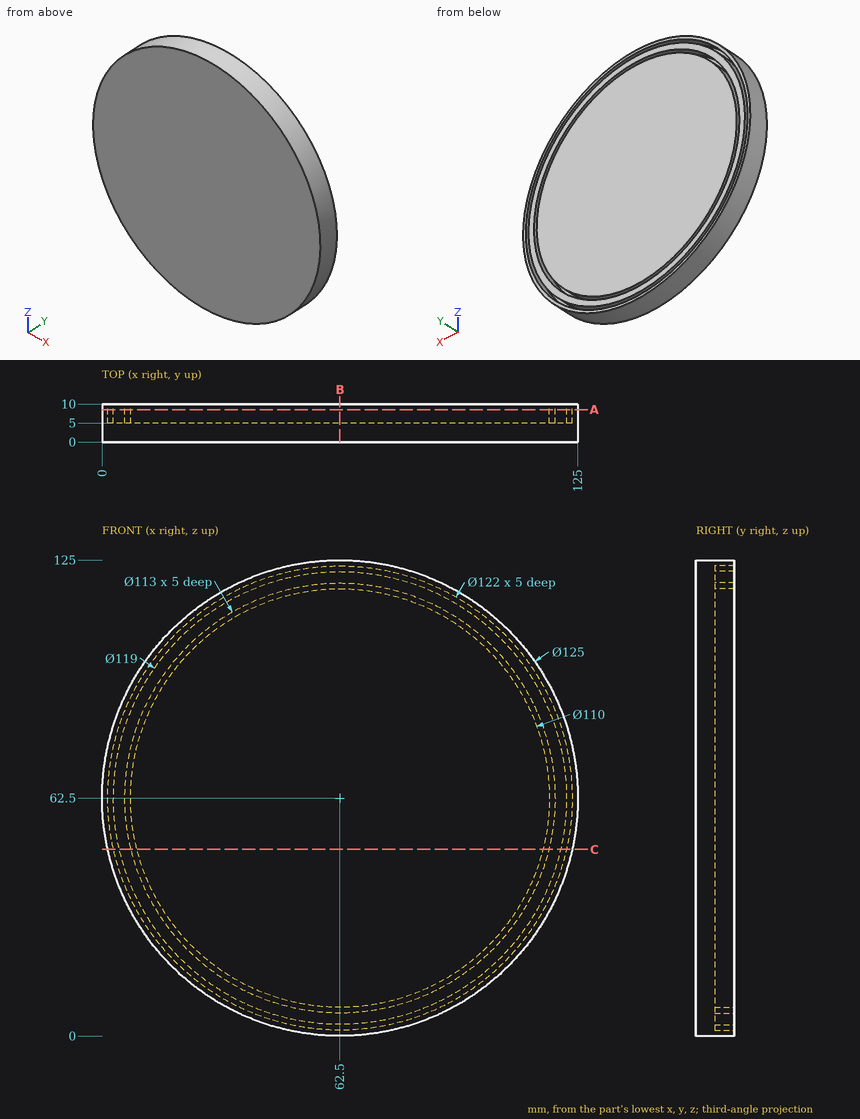
Answer from the drawing. Dimensions are ordinates in mm from the lowest x, y and z of the part. Round coordinates to 2 decimals unless told otherwise and drop trailing zeros. Loops run counter-clockwise (first coordinate to the right, second up) from the corner with the lowest first, then second, coordinate; pieces in that order, holes last. Notation, with made-up numbers: (55, 27.5) - (96, 27.5) arc R8 ccw to (96, 34.5) - close; hole circle Ø9 at (-4.5, 49.25). An arc over 180 degrees is marked (long way). One line per item, written item: value.
Q1. Find section C-C on z = 49. Give the vertices of the cut face in (x, y), and give its area (3 significant figures).
Check values:
outline: (1.48, 0) - (123.52, 0) - (123.52, 10) - (121.99, 10) - (121.99, 5) - (120.45, 5) - (120.45, 10) - (117.36, 10) - (117.36, 5) - (115.82, 5) - (115.82, 10) - (9.18, 10) - (9.18, 5) - (7.64, 5) - (7.64, 10) - (4.55, 10) - (4.55, 5) - (3.01, 5) - (3.01, 10) - (1.48, 10) - close
area: 1,190 mm2
Q2. Straight lines are drawn through the part: probe 1 along X at (y, z) = (7.25, 62.5); probe 2 along Z at (x, y) = (61.5, 9); probe 3 along X at (y, z) = (6.75, 47.5). For each, find the intervals that lie inside material, in ascending order.
Check values:
probe 1: 0 to 1.5, 3 to 6, 7.5 to 117.5, 119 to 122, 123.5 to 125
probe 2: 0.01 to 1.51, 3.01 to 6.01, 7.51 to 117.49, 118.99 to 121.99, 123.49 to 124.99
probe 3: 1.83 to 3.37, 4.92 to 8.03, 9.58 to 115.42, 116.97 to 120.08, 121.63 to 123.17
Q3. Each of these flat-tipped pins is pushed along its axis until it touches: pin 1 Ø1 at (x, y) = (70, 7.5) entering from +Z; pin 2 Ø1 at (y, z) = (6, 71) entering from -X; pin 3 Ø2 at (y, z) = (5.5, 106.5) entering from +X. Where does it stop, or does it pass through?
Check values:
pin 1: z = 124.61
pin 2: x = 0.51
pin 3: x = 107.86
Q4. Find section A-A on y = 8.5. Give the vertices of the cut face in (x, z).
Check values:
outline: circle Ø125 at (62.5, 62.5); circle Ø119 at (62.5, 62.5); circle Ø110 at (62.5, 62.5); hole circle Ø122 at (62.5, 62.5); hole circle Ø113 at (62.5, 62.5)
Q5. Find section B-B on x = 62.5. Give the vertices of the cut face in (y, z).
Check values:
outline: (0, 0) - (10, 0) - (10, 1.5) - (5, 1.5) - (5, 3) - (10, 3) - (10, 6) - (5, 6) - (5, 7.5) - (10, 7.5) - (10, 117.5) - (5, 117.5) - (5, 119) - (10, 119) - (10, 122) - (5, 122) - (5, 123.5) - (10, 123.5) - (10, 125) - (0, 125) - close
